For this review, use the dimensioned drawing (mm, ordinates from the lowest corner) and the shaded views. A direction names the side the tool comes from. Round coordinates to 2 decimals unless told otherwise and drop trailing zeros. Write each loop counter-clockwise with the first axis right and the second up, starting at its lowest first coordinate (ties: lowest second). Pieces come first, ordered by that corner, then holes. Notation, with made-up numbers: M 14.5,68.5 L 70.5,68.5 A30 cw 70.5,91.5 Z; hole C -2.5,39.5 d2. An arc over 180 degrees is marked long. One line per question, with ' | ' between items.
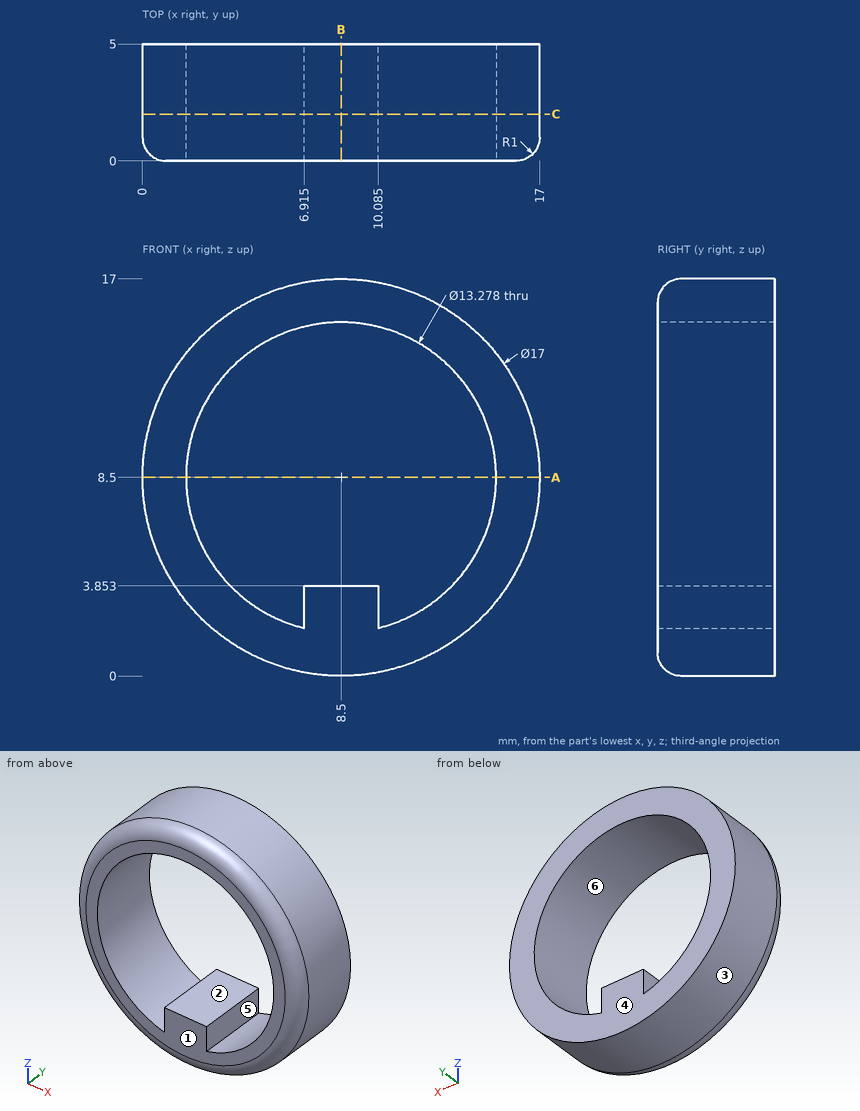
Item 1: Take a section at C-C (y = 2). Write out the cut boundary in (x, z) (3 decimals).
Results:
outline: C 8.5,8.5 d17; hole M 6.915,2.053 L 6.915,3.853 L 10.085,3.853 L 10.085,2.053 A6.639 ccw long Z
Item 2: Take a section at A-A (z = 8.5). Write out the cut boundary in (x, y), then the cut area to 3 significant figures.
Results:
outline: M 0,1 A1 ccw 1,0 L 1.86,0 L 1.86,5 L 0,5 Z; M 15.14,0 L 16,0 A1 ccw 17,1 L 17,5 L 15.14,5 Z | area: 18.2 mm2
Item 3: Take a section at B-B (x = 8.5). Write out the cut boundary in (y, z), then the cut area to 3 significant figures.
Results:
outline: M 0,1 A1 ccw 1,0 L 5,0 L 5,3.85 L 0,3.85 Z; M 0,15.14 L 5,15.14 L 5,17 L 1,17 A1 ccw 0,16 Z | area: 28.1 mm2
Item 4: Insertion check: pin 1 Ø3 at (y, z) = (3, 15) entering from +X; pin 2 Ø1.4 at (y, z) = (1.5, 2.5) entering from +X; pin 3 Ø0.9 at (y, z) = (1.5, 3) entering from -X. Each pin has a flat end and moves straight along its axis. Give the tip position at first contact, or say it passes through.
Results:
pin 1: x = 15.37 | pin 2: x = 15.15 | pin 3: x = 1.66
Item 5: Machinability: for the marked faces 1 and 2, which of the approach directions +Z, -Z, +X, -X, +Y, -Y give a long, thin tool a straight path to every point of the face, cutting with its end or side? Answer none if there is none.
Results:
face 1: +Z, -Z, +X, -X, -Y | face 2: +Y, -Y
Item 6: Mouldability with a two-part tool opening along X and no side actions: class the marked faces 3, 4, 5 and 6 as +X half, -X half, draft (parallel to the pull), parting line (faces both ways), or undercut.
Results:
face 3: parting line | face 4: draft | face 5: undercut | face 6: undercut
Item 7: To check wall thickness, follow line 1 along X through (y, z) = (2.8, 8.5); line 2 along X through (y, z) = (2.65, 2.75) (1 decimal); line 3 along X through (y, z) = (4.4, 3.25) (3 decimals). State the ranges of each line that lie inside material, in increasing order. Write a range as from..to.
Results:
line 1: 0..1.86, 15.14..17 | line 2: 2.2..5.2, 6.9..10.1, 11.8..14.8 | line 3: 1.815..4.436, 6.915..10.085, 12.564..15.185
